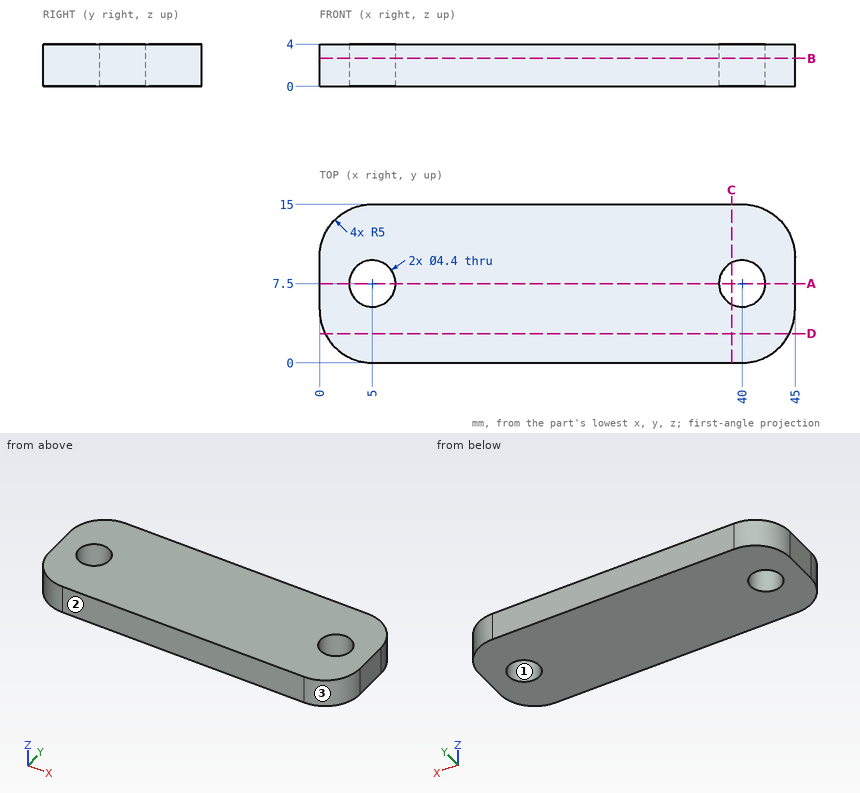
Check sheet for the drawn part. Datum: minimum x, y, z corner. Units: mm. Give positions to 0.01 mm unless a question says otherwise; leave off trailing zeros. Order: outer loops, then holes, each group sorted by start corner. A loop starts at its lowest first (then second) coordinate and runs counter-clockwise, first axis right, second up. Notation, with made-up numbers: (-5.75, 45.25) - (47.25, 45.25) arc R24 ccw to (47.25, 81.25) - close; hole circle Ø10 at (-13.75, 10). An arc over 180 degrees is marked (long way). Answer in a Markdown table with one row per item. Add a question column.
Q1. Mould release check, pull along X, two halves, no side actions. Record for the marked faces 1, 2 and 3: pulls with the +X half, pulls with the -X half, needs draft (parallel to the pull), parting line crosses it, or undercut.
Q2. Gauge pin test, flat ends, axial feed: pin 1 (3.5 mm diameter, centred on x = 40, y = 7.5, fed in from -Z); pin 2 (1 mm diameter, centred on y = 4, z = 3.5, fed in from -X). Record the tip position at first contact, or that the pin passes through.
Q3. Material ranges on probe 1 along Y at (x, z) = (5, 0.9); probe 2 along X at (y, z) = (7, 1.2); probe 3 along X at (y, z) = (6.5, 2.4), recorded low to high. Write a range as from..to.
Q4. Cross-section at D-D, the plane y = 2.75. Enter the section's corners in (x, z), then the cut area to 3 significant figures.
Q5. Cross-section at B-B, the plane z = 2.65. Enter the section's corners in (x, y).
Q6. Cross-section at A-A, the plane y = 7.5. Enter the section's corners in (x, z), then the cut area to 3 significant figures.
Q7. Cross-section at C-C, the plane x = 39. Enter the section's corners in (y, z).
Check values:
| question | item | result |
|---|---|---|
| 1 | face 1 | undercut |
| 1 | face 2 | needs draft |
| 1 | face 3 | pulls with the +X half |
| 2 | pin 1 | passes through |
| 2 | pin 2 | stops at x = 0.03 |
| 3 | probe 1 | y = 0..5.3, 9.7..15 |
| 3 | probe 2 | x = 0..2.86, 7.14..37.86, 42.14..45 |
| 3 | probe 3 | x = 0..3.04, 6.96..38.04, 41.96..45 |
| 4 | outline | (0.53, 0) - (44.47, 0) - (44.47, 4) - (0.53, 4) - close |
| 4 | area | 176 mm^2 |
| 5 | outline | (0, 5) arc R5 ccw to (5, 0) - (40, 0) arc R5 ccw to (45, 5) - (45, 10) arc R5 ccw to (40, 15) - (5, 15) arc R5 ccw to (0, 10) - close; hole circle Ø4.4 at (5, 7.5); hole circle Ø4.4 at (40, 7.5) |
| 6 | outline | (0, 0) - (2.8, 0) - (2.8, 4) - (0, 4) - close; (7.2, 0) - (37.8, 0) - (37.8, 4) - (7.2, 4) - close; (42.2, 0) - (45, 0) - (45, 4) - (42.2, 4) - close |
| 6 | area | 145 mm^2 |
| 7 | outline | (0, 0) - (5.54, 0) - (5.54, 4) - (0, 4) - close; (9.46, 0) - (15, 0) - (15, 4) - (9.46, 4) - close |
